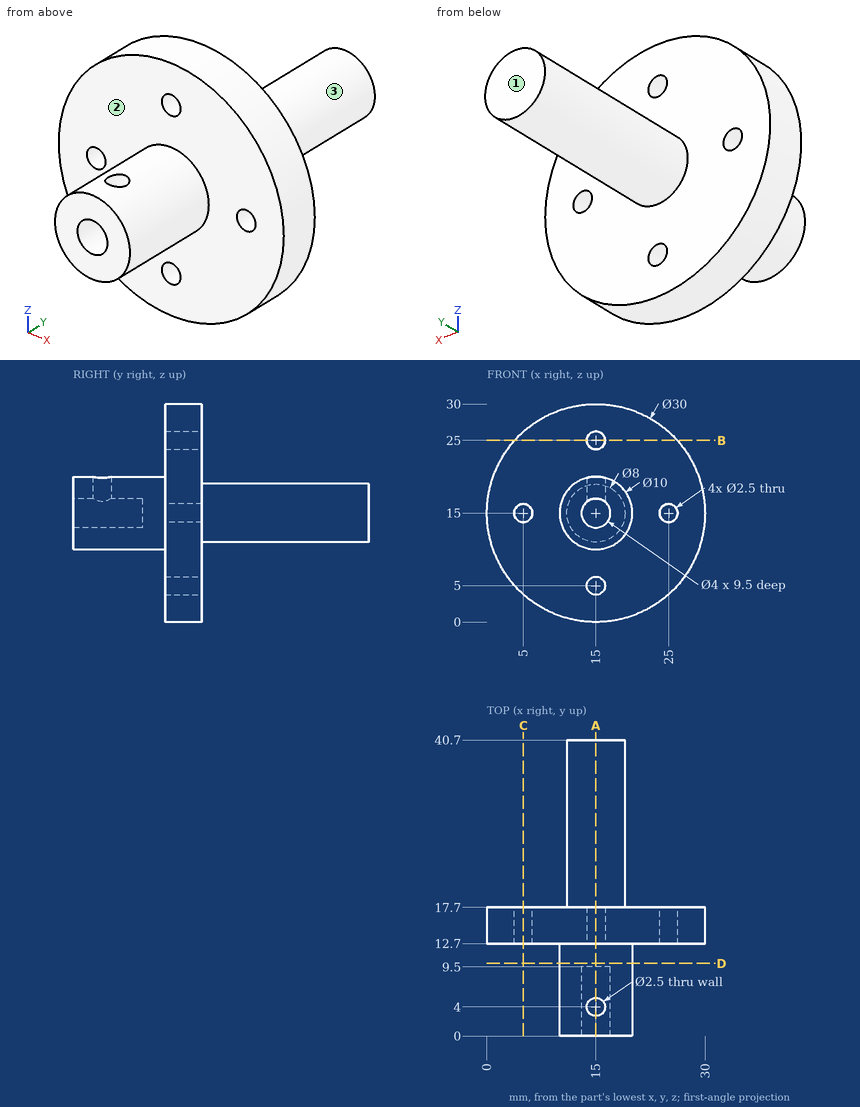
Part print with two shaded views. Sizes in mm from the minimum x, y, z corner. A direction names the side the tool comes from. Give positions to 0.01 mm unless a question says otherwise; leave off trailing zeros. Order: outer loops, then holes, each group sorted by start corner. A loop starts at its lowest first (then second) coordinate and runs counter-clockwise, first axis right, second up.
(1) Tool access for the marked faces 1, 2 and 3: list every direction of +Z, -Z, +X, -X, +Y, -Y with a clear straight run to the whole face (end or side of a thin tool).
(2) Saw through at D-D, the plane y = 10. Give the cut face in (x, z), then the cut area to 3 significant figures.
(3) Saw through at A-A, the plane x = 15. Give the cut face in (y, z), then the cut area to 4 significant figures.
(4) Drill centre lines: L1, parallel to Z at x = 15, y = 15.8; L2, parallel to Z at x = 15, y = 5.75; L3, parallel to X at y = 13.5, z = 15.75. Where is each one in solid material? Low to high.
(5) Flat gauge pins, fed straight in: pin 1 (3 mm diameter, centred on x = 11, z = 5, fed in from +Y); pin 2 (1.5 mm diameter, centred on x = 5, z = 15, fed in from +Y); pin 3 (1.5 mm diameter, centred on x = 22, y = 17.5, fed in from -Z); pin 4 (1.5 mm diameter, centred on x = 9, y = 13, fed in from -Z). Where does each tip first touch, or does it go through?
(6) Saw through at B-B, the plane z = 25. Give the cut face in (x, y).
(7) Saw through at C-C, the plane x = 5. Give the cut face in (y, z).
Results found:
1. face 1: +Z, -Z, +X, -X, +Y
1. face 2: -Y
1. face 3: +Y
2. outline: circle Ø10 at (15, 15)
2. area: 78.5 mm2
3. outline: (0, 10) - (12.7, 10) - (12.7, 6.25) - (17.7, 6.25) - (17.7, 11) - (40.7, 11) - (40.7, 19) - (17.7, 19) - (17.7, 23.75) - (12.7, 23.75) - (12.7, 20) - (5.25, 20) - (5.25, 17) - (9.5, 17) - (9.5, 13) - (0, 13) - close; (0, 17) - (2.75, 17) - (2.75, 20) - (0, 20) - close; (12.7, 0) - (17.7, 0) - (17.7, 3.75) - (12.7, 3.75) - close; (12.7, 26.25) - (17.7, 26.25) - (17.7, 30) - (12.7, 30) - close
3. area: 390.5 mm2
4. L1: z = 0 to 3.75, 6.25 to 23.75, 26.25 to 30
4. L2: z = 10 to 13, 17 to 20
4. L3: x = 0.02 to 4, 6 to 24, 26 to 29.98
5. pin 1: stops at y = 17.7
5. pin 2: passes through
5. pin 3: stops at z = 1.36
5. pin 4: stops at z = 0.95
6. outline: (3.82, 12.7) - (13.75, 12.7) - (13.75, 17.7) - (3.82, 17.7) - close; (16.25, 12.7) - (26.18, 12.7) - (26.18, 17.7) - (16.25, 17.7) - close
7. outline: (12.7, 3.82) - (17.7, 3.82) - (17.7, 13.75) - (12.7, 13.75) - close; (12.7, 16.25) - (17.7, 16.25) - (17.7, 26.18) - (12.7, 26.18) - close
